Autodesk Inventor part; units mm, degrees
ref_plane "YZ Plane" through (0, 0, 0) normal (1, 0, 0) x (0, 1, 0)
ref_plane "XZ Plane" through (0, 0, 0) normal (0, 1, 0) x (-1, 0, 0)
ref_plane "XY Plane" through (0, 0, 0) normal (0, 0, 1) x (1, 0, 0)
sketch "Sketch1" plane through (0, 0, 0) normal (0, 1, 0) x (-1, 0, 0)
  line L0 (10, 40) -> (-10, 40)
  line L1 (-10, 40) -> (-10, -40)
  line L2 (-10, -40) -> (10, -40)
  line L3 (10, -40) -> (10, 40)
  point P0 (0, 0)
  point P1 (10, 0)
  point P2 (0, -40)
  dimension "d0" = 80
  dimension "d1" = 20
extrude "MainCore" add sketch "Sketch1" along normal blind 70
sketch "Sketch3" plane through (0, 70, 0) normal (0, 1, 0) x (1, 0, 0)
  line L0 (-10, -10) -> (10, -10)
  line L1 (10, -10) -> (10, 10)
  line L2 (10, 10) -> (-10, 10)
  line L3 (-10, 10) -> (-10, -10)
  line L4 (-10, 40) -> (-10, -40)
  line L5 (-10, -30) -> (10, -30)
  line L6 (10, -30) -> (10, -10)
  line L7 (10, -10) -> (-10, -10)
  line L8 (-10, -10) -> (-10, -30)
  line L9 (-10, 10) -> (10, 10)
  line L10 (10, 10) -> (10, 30)
  line L11 (10, 30) -> (-10, 30)
  line L12 (-10, 30) -> (-10, 10)
  point P0 (0, 0)
  point P1 (-10, 0)
  point P2 (0, 10)
  point P3 (0, -10)
  point P4 (0, 10)
  dimension "d4" = 20
  dimension "d5" = 20
  dimension "d6" = 20
extrude "Windows" cut sketch "Sketch3" against normal blind 50 contours L0 L6 L5 L4 | L4 L11 L10 L2
fillet "Outer corners" radius 2.4 2 edges at (0, 0, -40) (0, 0, 40)
fillet "Fillet2" radius 1 4 edges at (0, 20, 10) (0, 20, 30) (0, 20, -10) (0, 20, -30)
equation "\"d0\" = coreWidth"
equation "\"d1\" = coreDepth"
equation "\"d4\" = coreLegWidthInner"
equation "\"d5\" = -0.5 * coreLegWidthInner + 0.5 * coreWidthInner"
equation "\"d6\" = -0.5 * coreLegWidthInner + 0.5 * coreWidthInner"
equation "\"d9\" = 0.03 * coreWidth"
equation "\"d10\" = 0.025 * coreWidthInner - 0.025 * coreLegWidthInner"
equation "\"coreWidth\" = 80"
equation "\"coreDepth\" = 20"
equation "\"coreLegWidthInner\" = 20"
equation "\"wallThick\" = 1"
equation "\"extDepth\" = 31.8"
equation "\"WireDia\" = 1.2"
equation "\"Airgap\" = 0.24"
properties part number "coil 55_28_21-02"
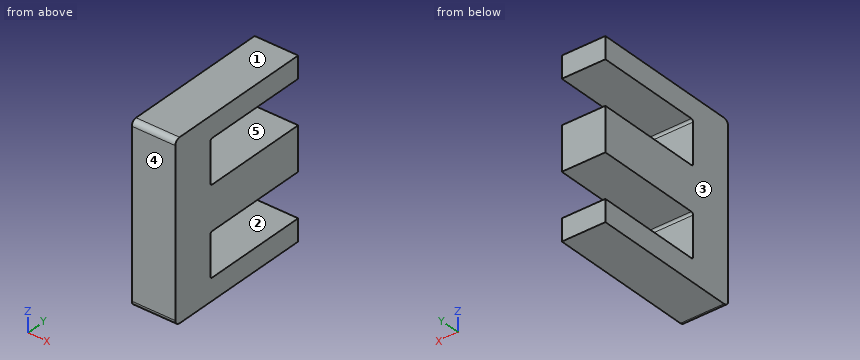
Part model, mm, in its own coordinate system. Face numbers are marked on the shaded views. A direction names the side the tool comes from. Coordinates: 2 decimals unless noted, no trailing zeros. Write each loop counter-clockwise with the first axis right and the second up, starting at its lowest first coordinate (ties: lowest second). Pieces come first, ordered by that corner, then holes.
Item 1: Slice it at B-B (x = -4.5). Write the cut outline in (y, z), and give its area (3 significant figures).
Item 2: Slice it at A-A (y = 52). Write the cut outline in (x, z), and give its area (3 significant figures).
Item 3: Probe line 1 (Z direction, x = 3.75, y = 62.5); line 2 (Y direction, x = 5.25, z = -17.5). List the from-to ranges inside material, lowest first.
Item 4: Which spindle directions (+Z, -Z, +X, -X, +Y, -Y) get a long thin tool onto all of the face, cutting with end or side? Do the marked faces 4 and 5. Say none if no direction does.
Item 5: Pin check, flat tips, straight feed: pin 1 (5.5 mm diameter, centred on x = -3, z = -20, fed in from +Y); pin 2 (12 mm diameter, centred on y = 26.5, z = 23.5, fed in from +X). Stop position of each tip, or through.
Item 6: Slice it at C-C (z = -24). Write the cut outline in (x, y).
Item 7: Mould opens along Z. For the marked faces 1, 2 and 3 say: released by +Z, released by -Z, zero draft, split by the parting line, or undercut.
Results found:
1. outline: (0, -37.6) arc R2.4 ccw to (2.4, -40) - (70, -40) - (70, -30) - (21, -30) arc R1 cw to (20, -29) - (20, -11) arc R1 cw to (21, -10) - (70, -10) - (70, 10) - (21, 10) arc R1 cw to (20, 11) - (20, 29) arc R1 cw to (21, 30) - (70, 30) - (70, 40) - (2.4, 40) arc R2.4 ccw to (0, 37.6) - close
1. area: 3,600 mm2
2. outline: (-10, -40) - (10, -40) - (10, -30) - (-10, -30) - close; (-10, -10) - (10, -10) - (10, 10) - (-10, 10) - close; (-10, 30) - (10, 30) - (10, 40) - (-10, 40) - close
2. area: 800 mm2
3. line 1: z = -40 to -30, -10 to 10, 30 to 40
3. line 2: y = 0 to 20
4. face 4: +Z, -Z, +X, -X, -Y
4. face 5: +X, -X, +Y
5. pin 1: stops at y = 20
5. pin 2: passes through
6. outline: (-10, 0) - (10, 0) - (10, 20) - (-10, 20) - close
7. face 1: released by +Z
7. face 2: undercut
7. face 3: zero draft
